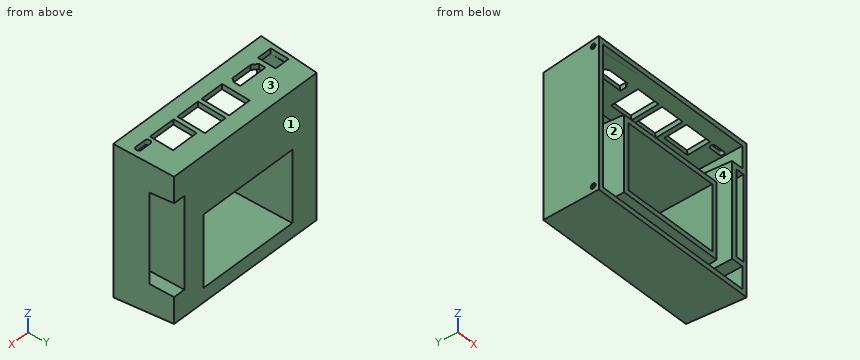
```python
from build123d import *

# Parameters (mm, degrees)
SKETCH2_W                                         = 103
SKETCH2_H                                         = 90
SKETCH2_W_2                                       = 4.981131341
SKETCH2_H_2                                       = 51.379447355
SKETCH2_W_3                                       = 58.371562284
SKETCH2_H_3                                       = 39.434223375
BOSS_EXTRUDE2_DEPTH                               = 35
BOSS_EXTRUDE2_TAPER                               = 3
SHELL2_OUTLINE_W                                  = 67.733894234
SHELL2_OUTLINE_H                                  = 48.796555325
SHELL2_DEPTH                                      = 32
SHELL2_DRAFT                                      = 3
SKETCH11_W                                        = 8.997468353
SKETCH11_H                                        = 10.72090286
CUT_EXTRUDE2_DEPTH                                = 3
CUT_EXTRUDE2_DRAFT                                = -3
SKETCH11_W_2                                      = 14.518642115
SKETCH11_H_2                                      = 16.642925392
CUT_EXTRUDE2_PROFILE_2_DEPTH                      = 3
CUT_EXTRUDE2_PROFILE_2_DRAFT                      = -3
SKETCH11_W_3                                      = 14.620886073
CUT_EXTRUDE2_PROFILE_3_DEPTH                      = 3
CUT_EXTRUDE2_PROFILE_3_DRAFT                      = -3
SKETCH11_W_4                                      = 16.665765244
SKETCH11_H_3                                      = 13.8861218
CUT_EXTRUDE2_PROFILE_4_DEPTH                      = 3
CUT_EXTRUDE2_PROFILE_4_DRAFT                      = -3
CUT_EXTRUDE2_PROFILE_5_DEPTH                      = 3
CUT_EXTRUDE2_PROFILE_5_DRAFT                      = -3
CUT_EXTRUDE2_PROFILE_6_DEPTH                      = 3
CUT_EXTRUDE2_PROFILE_6_DRAFT                      = -3
CSK_FOR_0_FLAT_HEAD_MACHINE_SCREW_100_D           = 1.778
CSK_FOR_0_FLAT_HEAD_MACHINE_SCREW_100_CSINK_D     = 3.0226
CSK_FOR_0_FLAT_HEAD_MACHINE_SCREW_100_CSINK_ANGLE = 100
CSK_FOR_0_FLAT_HEAD_MACHINE_SCREW_2_D             = 1.778
CSK_FOR_0_FLAT_HEAD_MACHINE_SCREW_2_CSINK_D       = 3.0226
CSK_FOR_0_FLAT_HEAD_MACHINE_SCREW_2_CSINK_ANGLE   = 100
DRAFT4_START                                      = 5
DRAFT4_DEPTH                                      = 19


with BuildPart() as part:
    # Sketch2 → Boss-Extrude2 (new body)
    with BuildSketch(Plane(origin=(0, 0, 0), x_dir=(1, 0, 0), z_dir=(0, 1, 0))):
        with Locations((51.5, 0)):
            Rectangle(SKETCH2_W, SKETCH2_H)
        with Locations((98.329809834, -0.07834477)):
            Rectangle(SKETCH2_W_2, SKETCH2_H_2, mode=Mode.SUBTRACT)
        with Locations((49.815754183, 13.061230018)):
            Rectangle(SKETCH2_W_3, SKETCH2_H_3, mode=Mode.SUBTRACT)
    extrude(amount=BOSS_EXTRUDE2_DEPTH, taper=BOSS_EXTRUDE2_TAPER)


with BuildPart() as shell2_tool:
    # Shell2: read off the stored shape, not the designer's step
    # Shell2 outline → Shell2 (with draft: the straight prism first)
    with BuildSketch(Plane(origin=(0, 32, 0), x_dir=(1, 0, 0), z_dir=(0, 1, 0))):
        Polygon((98.318834025, -30.449234423), (91.158078188, -30.449234423), (91.158078188, 30.292544882), (98.318834025, 30.292544882), (98.318834025, 40.318834025), (4.681165975, 40.318834025), (4.681165975, -40.318834025), (98.318834025, -40.318834025), align=None)
        with Locations((49.815754183, 13.061230019)):
            Rectangle(SHELL2_OUTLINE_W, SHELL2_OUTLINE_H, mode=Mode.SUBTRACT)
    extrude(amount=-SHELL2_DEPTH)
    # Shell2: the draft: its side faces are tilted about the plane it starts from
    shell2_sides = [shell2_tool.faces().sort_by_distance(p)[0] for p in [
        (94.738456106, 16, 30.449234423),
        (91.158078188, 16, 0.07834477),
        (94.738456107, 16, -30.292544882),
        (98.318834025, 16, -35.305689454),
        (51.5, 16, -40.318834025),
        (4.681165975, 16, 0),
        (51.5, 16, 40.318834025),
        (98.318834025, 16, 35.384034224),
        (15.948807066, 16, -13.061230018),
        (49.815754183, 16, -37.459507681),
        (83.6827013, 16, -13.061230018),
        (49.815754183, 16, 11.337047644),
    ]]
    draft(shell2_sides, Plane(origin=(0, 32, 0), x_dir=(1, 0, 0), z_dir=(0, 1, 0)), SHELL2_DRAFT)


with BuildPart() as part_1:
    add(part.part)

    # Shell2: cut by shell2_tool
    add(shell2_tool.part, mode=Mode.SUBTRACT)


with BuildPart() as cut_extrude2_tool:
    # Sketch11 → Cut-Extrude2 (with draft: the straight prism first)
    with BuildSketch(Plane(origin=(0, 2.351890424, 44.876742646), x_dir=(1, 0, 0), z_dir=(0, 0.0523359562429439, 0.998629534754574))):
        with Locations((7.959003718, 11.806398056)):
            Rectangle(SKETCH11_W, SKETCH11_H)
    extrude(amount=-CUT_EXTRUDE2_DEPTH)
    # Cut-Extrude2: the draft: its side faces are tilted about the plane it starts from
    cut_extrude2_sides = [cut_extrude2_tool.faces().sort_by_distance(p)[0] for p in [
        (3.460269541, 14.063604287, 42.760899212),
        (7.959003718, 8.710499169, 43.041443563),
        (12.457737894, 14.063604287, 42.760899212),
        (7.959003718, 19.416709405, 42.48035486),
    ]]
    draft(cut_extrude2_sides, Plane(origin=(0, 2.351890424, 44.876742646), x_dir=(1, 0, 0), z_dir=(0, 0.0523359562429439, 0.998629534754574)), CUT_EXTRUDE2_DRAFT)


with BuildPart() as part_2:
    add(part_1.part)

    # Cut-Extrude2: cut by cut_extrude2_tool
    add(cut_extrude2_tool.part, mode=Mode.SUBTRACT)


with BuildPart() as cut_extrude2_profile_2_tool:
    # Sketch11 → Cut-Extrude2 profile 2 (with draft: the straight prism first)
    with BuildSketch(Plane(origin=(0, 2.351890424, 44.876742646), x_dir=(1, 0, 0), z_dir=(0, 0.0523359562429439, 0.998629534754574))):
        with Locations((44.664584839, 14.767409322)):
            Rectangle(SKETCH11_W_2, SKETCH11_H_2)
    extrude(amount=-CUT_EXTRUDE2_PROFILE_2_DEPTH)
    # Cut-Extrude2 profile 2: the draft: its side faces are tilted about the plane it starts from
    cut_extrude2_profile_2_sides = [cut_extrude2_profile_2_tool.faces().sort_by_distance(p)[0] for p in [
        (37.405263781, 17.02055759, 42.605931856),
        (44.664584839, 8.710499169, 43.041443563),
        (51.923905896, 17.02055759, 42.605931856),
        (44.664584839, 25.330616011, 42.170420148),
    ]]
    draft(cut_extrude2_profile_2_sides, Plane(origin=(0, 2.351890424, 44.876742646), x_dir=(1, 0, 0), z_dir=(0, 0.0523359562429439, 0.998629534754574)), CUT_EXTRUDE2_PROFILE_2_DRAFT)


with BuildPart() as part_3:
    add(part_2.part)

    # Cut-Extrude2 profile 2: cut by cut_extrude2_profile_2_tool
    add(cut_extrude2_profile_2_tool.part, mode=Mode.SUBTRACT)


with BuildPart() as cut_extrude2_profile_3_tool:
    # Sketch11 → Cut-Extrude2 profile 3 (with draft: the straight prism first)
    with BuildSketch(Plane(origin=(0, 2.351890424, 44.876742646), x_dir=(1, 0, 0), z_dir=(0, 0.0523359562429439, 0.998629534754574))):
        with Locations((61.48371602, 14.767409322)):
            Rectangle(SKETCH11_W_3, SKETCH11_H_2)
    extrude(amount=-CUT_EXTRUDE2_PROFILE_3_DEPTH)
    # Cut-Extrude2 profile 3: the draft: its side faces are tilted about the plane it starts from
    cut_extrude2_profile_3_sides = [cut_extrude2_profile_3_tool.faces().sort_by_distance(p)[0] for p in [
        (54.173272984, 17.02055759, 42.605931856),
        (61.483716021, 8.710499169, 43.041443563),
        (68.794159057, 17.02055759, 42.605931856),
        (61.483716021, 25.330616011, 42.170420148),
    ]]
    draft(cut_extrude2_profile_3_sides, Plane(origin=(0, 2.351890424, 44.876742646), x_dir=(1, 0, 0), z_dir=(0, 0.0523359562429439, 0.998629534754574)), CUT_EXTRUDE2_PROFILE_3_DRAFT)


with BuildPart() as part_4:
    add(part_3.part)

    # Cut-Extrude2 profile 3: cut by cut_extrude2_profile_3_tool
    add(cut_extrude2_profile_3_tool.part, mode=Mode.SUBTRACT)


with BuildPart() as cut_extrude2_profile_4_tool:
    # Sketch11 → Cut-Extrude2 profile 4 (with draft: the straight prism first)
    with BuildSketch(Plane(origin=(0, 2.351890424, 44.876742646), x_dir=(1, 0, 0), z_dir=(0, 0.0523359562429439, 0.998629534754574))):
        with Locations((79.478652726, 13.389007526)):
            Rectangle(SKETCH11_W_4, SKETCH11_H_3)
    extrude(amount=-CUT_EXTRUDE2_PROFILE_4_DEPTH)
    # Cut-Extrude2 profile 4: the draft: its side faces are tilted about the plane it starts from
    cut_extrude2_profile_4_sides = [cut_extrude2_profile_4_tool.faces().sort_by_distance(p)[0] for p in [
        (71.145770104, 15.644044846, 42.678071832),
        (79.478652726, 8.710499169, 43.041443563),
        (87.811535348, 15.644044846, 42.678071832),
        (79.478652726, 22.577590522, 42.3147001),
    ]]
    draft(cut_extrude2_profile_4_sides, Plane(origin=(0, 2.351890424, 44.876742646), x_dir=(1, 0, 0), z_dir=(0, 0.0523359562429439, 0.998629534754574)), CUT_EXTRUDE2_PROFILE_4_DRAFT)


with BuildPart() as part_5:
    add(part_4.part)

    # Cut-Extrude2 profile 4: cut by cut_extrude2_profile_4_tool
    add(cut_extrude2_profile_4_tool.part, mode=Mode.SUBTRACT)


with BuildPart() as cut_extrude2_profile_5_tool:
    # Sketch11 → Cut-Extrude2 profile 5 (with draft: the straight prism first)
    with BuildSketch(Plane(origin=(0, 2.351890424, 44.876742646), x_dir=(1, 0, 0), z_dir=(0, 0.0523359562429439, 0.998629534754574))):
        Polygon((18.38788749, 7.26277732), (31.066138351, 7.26277732), (33.008773563, 9.713269403), (33.008773563, 13.389007526), (15.218324775, 13.389007526), (15.218324775, 9.713269403), align=None)
    extrude(amount=-CUT_EXTRUDE2_PROFILE_5_DEPTH)
    # Cut-Extrude2 profile 5: the draft: its side faces are tilted about the plane it starts from
    cut_extrude2_profile_5_sides = [cut_extrude2_profile_5_tool.faces().sort_by_distance(p)[0] for p in [
        (24.727012921, 9.526210425, 42.998693948),
        (32.037455957, 10.74977731, 42.934569524),
        (33.008773563, 13.80869452, 42.774258466),
        (24.113549169, 15.644044846, 42.678071832),
        (15.218324775, 13.80869452, 42.774258466),
        (16.803106133, 10.74977731, 42.934569524),
    ]]
    draft(cut_extrude2_profile_5_sides, Plane(origin=(0, 2.351890424, 44.876742646), x_dir=(1, 0, 0), z_dir=(0, 0.0523359562429439, 0.998629534754574)), CUT_EXTRUDE2_PROFILE_5_DRAFT)


with BuildPart() as part_6:
    add(part_5.part)

    # Cut-Extrude2 profile 5: cut by cut_extrude2_profile_5_tool
    add(cut_extrude2_profile_5_tool.part, mode=Mode.SUBTRACT)


with BuildPart() as cut_extrude2_profile_6_tool:
    # Sketch11 → Cut-Extrude2 profile 6 (with draft: the straight prism first)
    with BuildSketch(Plane(origin=(0, 2.351890424, 44.876742646), x_dir=(1, 0, 0), z_dir=(0, 0.0523359562429439, 0.998629534754574))):
        with BuildLine():
            ThreePointArc((91.287829939, 9.713269403), (89.654168551, 8.079608014), (91.287829939, 6.445946626))
            Line((91.287829939, 6.445946626), (97.320223494, 6.445946626))
            ThreePointArc((97.320223494, 6.445946626), (98.953884882, 8.079608014), (97.320223494, 9.713269403))
            Line((97.320223494, 9.713269403), (91.287829939, 9.713269403))
        make_face()
    extrude(amount=-CUT_EXTRUDE2_PROFILE_6_DEPTH)
    # Cut-Extrude2 profile 6: the draft: its side faces are tilted about the plane it starts from
    cut_extrude2_profile_6_sides = [cut_extrude2_profile_6_tool.faces().sort_by_distance(p)[0] for p in [
        (94.304026716, 11.973344194, 42.870445101),
        (89.654168551, 10.341921681, 42.955944332),
        (94.304026716, 8.710499169, 43.041443563),
        (98.953884882, 10.341921681, 42.955944332),
    ]]
    draft(cut_extrude2_profile_6_sides, Plane(origin=(0, 2.351890424, 44.876742646), x_dir=(1, 0, 0), z_dir=(0, 0.0523359562429439, 0.998629534754574)), CUT_EXTRUDE2_PROFILE_6_DRAFT)


with BuildPart() as part_7:
    add(part_6.part)

    # Cut-Extrude2 profile 6: cut by cut_extrude2_profile_6_tool
    add(cut_extrude2_profile_6_tool.part, mode=Mode.SUBTRACT)

    # CSK for _0 Flat Head Machine Screw _100 (through all)
    with Locations(Plane(origin=(0.188541787, 3.597591615, -41), x_dir=(-0.052335956243, -0.998629534755, 0), z_dir=(-0.998629534755, 0.052335956243, 0))):
        with Locations((0, 0), (0.002528755, 82)):
            CounterSinkHole(CSK_FOR_0_FLAT_HEAD_MACHINE_SCREW_100_D / 2, CSK_FOR_0_FLAT_HEAD_MACHINE_SCREW_100_CSINK_D / 2, counter_sink_angle=CSK_FOR_0_FLAT_HEAD_MACHINE_SCREW_100_CSINK_ANGLE)

    # CSK for _0 Flat Head Machine Screw _ 2 (through all)
    with Locations(Plane(origin=(0.188541787, 3.597591615, -41), x_dir=(-0.052335956243, -0.998629534755, 0), z_dir=(-0.998629534755, 0.052335956243, 0))):
        with Locations((0, 0), (0.002528755, 82)):
            CounterSinkHole(CSK_FOR_0_FLAT_HEAD_MACHINE_SCREW_2_D / 2, CSK_FOR_0_FLAT_HEAD_MACHINE_SCREW_2_CSINK_D / 2, counter_sink_angle=CSK_FOR_0_FLAT_HEAD_MACHINE_SCREW_2_CSINK_ANGLE)

    # Draft4: read off the stored shape, not the designer's step
    # Draft4 outline → Draft4 (add)
    with BuildSketch(Plane(origin=(0, 0, 0), x_dir=(1, 0, 0), z_dir=(0, 0.9986295347545739, -0.052335956242943814)).offset(DRAFT4_START)):
        Polygon((51.923905896, -44.938329064), (51.766682558, -41.938329064), (51.714317363, -44.938329064), align=None)
        Polygon((87.65431201, -41.938329064), (87.601946816, -44.938329064), (87.811535348, -44.938329064), align=None)
        Polygon((68.636935719, -41.938329064), (68.584570525, -44.938329064), (68.794159057, -44.938329064), align=None)
        Polygon((32.799185031, -44.938329064), (33.008773563, -44.938329064), (32.851550226, -41.938329064), align=None)
    extrude(amount=DRAFT4_DEPTH)


solid = part_7.part
```
The listing builds one solid part. Answer for the finished solid, in the listing's coordinates (mm). Face numbers are marked on the shaded views. Round coordinates to 2 decimals unless told otherwise and drop trailing zeros. Answer as CSV lines item,"result".
Q1. Consider line 1 (Z direction, x = 74.5, y = 20.5); line 2 (Z direction, x = 64, y = 24.5); line 3 (X direction, y = 12.5, z = -35.5). Determine where each line is inside the solid, lowest interval first. Write a range as from..to.
Computed values:
line 1,"z = -43.93..-40.92, -36.86..-33.85, 7.73..10.73"
line 2,"z = -43.72..-40.71, -37.07..-34.06, 7.94..10.94"
line 3,"x = 0.66..3.66, 16.97..82.66, 99.34..102.34"
Q2. A cutting plane is placed at A-A on x = 61.5. Give the number of separate pieces and of enclosed holes in the cut face, plus the area to 3 significant figures.
Computed values:
separate pieces,"3"
enclosed holes,"0"
area,"466 mm^2"
Q3. For a pull along Z with two mould halves and no side action, classify the marked faces 1, 2, 3 and 4 as +Z half, -Z half, draft (parallel to the pull), parting line (faces both ways), or undercut.
Computed values:
face 1,"draft"
face 2,"undercut"
face 3,"+Z half"
face 4,"undercut"
Q4. Given pin 1 (8 mm diameter, centred on y = 23.5, z = -9, fed in from +X); pin 2 (6 mm diameter, centred on x = 68.5, y = 13.5, fed in from -Z); pin 3 (5 mm diameter, centred on x = 71.5, y = 16, fed in from +Z), each flat-ended and moving along its own axis, determine where each tip first touches the part or whether it passes through.
Computed values:
pin 1,"stops at x = 101.98"
pin 2,"stops at z = -44.45"
pin 3,"stops at z = 44.29"
